```python
from build123d import *

# Parameters (mm, degrees)
SKETCH1_W                       = 180
SKETCH1_H                       = 60
BOSS_EXTRUDE1_DEPTH             = 15
CUT_EXTRUDE1_DEPTH              = 97.046863561
TAP_DRILL_FOR_M6X1_0_TAP1_D     = 5
TAP_DRILL_FOR_M6X1_0_TAP1_DEPTH = 9
TAP_DRILL_FOR_M6X1_0_TAP1_TIP   = 1.502151548
FILLET1_R                       = 25
TAP_DRILL_FOR_M6X1_0_TAP2_D     = 5
TAP_DRILL_FOR_M6X1_0_TAP2_DEPTH = 9
TAP_DRILL_FOR_M6X1_0_TAP2_TIP   = 1.502151548


with BuildPart() as part:
    # Sketch1 → Boss-Extrude1 (new body)
    with BuildSketch(Plane(origin=(0, 0, 0), x_dir=(1, 0, 0), z_dir=(0, 1, 0))):
        Rectangle(SKETCH1_W, SKETCH1_H)
    extrude(amount=BOSS_EXTRUDE1_DEPTH)

    # Sketch2 → Cut-Extrude1 (cut, through all)
    with BuildSketch(Plane(origin=(0, 15, 0), x_dir=(1, 0, 0), z_dir=(0, 1, 0))):
        with BuildLine():
            Line((-60, 17.5), (-23.75, 17.5))
            ThreePointArc((-23.75, 17.5), (-6.25, 0), (-23.75, -17.5))
            Line((-23.75, -17.5), (-60, -17.5))
            ThreePointArc((-60, -17.5), (-77.5, 0), (-60, 17.5))
        make_face()
        with BuildLine():
            Line((23.75, 17.5), (60, 17.5))
            ThreePointArc((60, 17.5), (77.5, 0), (60, -17.5))
            Line((60, -17.5), (23.75, -17.5))
            ThreePointArc((23.75, -17.5), (6.25, 0), (23.75, 17.5))
        make_face()
    extrude(amount=-CUT_EXTRUDE1_DEPTH, mode=Mode.SUBTRACT)

    # Tap Drill for M6x1.0 Tap1
    with Locations(Plane.XY.offset(30)):
        with Locations((60, 7.5), (-20, 7.5), (20, 7.5), (-60, 7.5)):
            Hole(TAP_DRILL_FOR_M6X1_0_TAP1_D / 2, depth=TAP_DRILL_FOR_M6X1_0_TAP1_DEPTH)
            with Locations((0, 0, -(TAP_DRILL_FOR_M6X1_0_TAP1_DEPTH + TAP_DRILL_FOR_M6X1_0_TAP1_TIP / 2))):  # 118° drill point
                Cone(0, TAP_DRILL_FOR_M6X1_0_TAP1_D / 2, TAP_DRILL_FOR_M6X1_0_TAP1_TIP, mode=Mode.SUBTRACT)

    # Fillet1
    fillet1_edges = [part.edges().sort_by_distance(p)[0] for p in [
        (-90, 7.5, -30),
        (90, 7.5, -30),
    ]]
    fillet(fillet1_edges, radius=FILLET1_R)

    # Tap Drill for M6x1.0 Tap2
    with Locations(Plane(origin=(0, 0, -30), x_dir=(-1, 0, 0), z_dir=(0, 0, -1))):
        with Locations((-45, 7.5), (-15, 7.5), (15, 7.5), (45, 7.5)):
            Hole(TAP_DRILL_FOR_M6X1_0_TAP2_D / 2, depth=TAP_DRILL_FOR_M6X1_0_TAP2_DEPTH)
            with Locations((0, 0, -(TAP_DRILL_FOR_M6X1_0_TAP2_DEPTH + TAP_DRILL_FOR_M6X1_0_TAP2_TIP / 2))):  # 118° drill point
                Cone(0, TAP_DRILL_FOR_M6X1_0_TAP2_D / 2, TAP_DRILL_FOR_M6X1_0_TAP2_TIP, mode=Mode.SUBTRACT)


solid = part.part
```
Read the model definition and answer for the solid it produces. Units are mm, in the model's axes. A direction names the side the tool comes from. Round coordinates to 2 decimals unless told otherwise and drop trailing zeros. Write each loop counter-clockwise with the first axis right and the second up, starting at its lowest first coordinate (ties: lowest second). Pieces come first, ordered by that corner, then holes. Notation, with made-up numbers: (33, 67) - (91, 67) arc R17 cw to (91, 84) - close; hole circle Ø6 at (-12.5, -38). An arc over 180 degrees is marked (long way). One line per item, written item: value.
Q1. For a pull along Y with two mould halves and no side action, classify faces 1 (the flat face through (-1, 15, 0)), 2 (the cylindrical face through (57.69, 6.54, 25.44)), 3 (the flat face through (-1, 7, -30)) as pulls with the +Y half, pulls with the -Y half, needs draft (parallel to the pull), parting line crosses it, or undercut.
The answers:
face 1: pulls with the +Y half
face 2: undercut
face 3: needs draft
Q2. Straight lines are drawn through the part: line 1 (X direction, y = 6, z = -1); line 2 (Z direction, x = -42.5, y = 1.75); line 3 (Y direction, x = -15, z = -23.75). For each, find the intervals that lie inside material, in ascending order. Write a range as from..to.
The answers:
line 1: x = -90..-77.47, -6.28..6.28, 77.47..90
line 2: z = -30..-17.5, 17.5..30
line 3: y = 0..5, 10..15
Q3. Find section C-C (x = -69). Determine the outline of the cut face in (y, z), and give its area (3 significant figures).
The answers:
outline: (0, -29.68) - (15, -29.68) - (15, -15.01) - (0, -15.01) - close; (0, 15.01) - (15, 15.01) - (15, 30) - (0, 30) - close
area: 445 mm2
Q4. Which of the six approach directions +Z, -Z, +X, -X, +Y, -Y give full straight-line access (tool end or side, diameter ignored) to faces 4 (the flat face through (-42, 8, 17.5)), 5 (the cylindrical face through (-18, 6, 25)), 6 (the cylindrical face through (-82.871, 7.605, -22.482)), 7 (the cylindrical face through (13, 6, -25))?
The answers:
face 4: +Y, -Y
face 5: +Z
face 6: -Z, -X, +Y, -Y
face 7: -Z
Q5. Find section B-B (z = 0). Determine the outline of the cut face in (x, y).
The answers:
outline: (-90, 0) - (-77.5, 0) - (-77.5, 15) - (-90, 15) - close; (-6.25, 0) - (6.25, 0) - (6.25, 15) - (-6.25, 15) - close; (77.5, 0) - (90, 0) - (90, 15) - (77.5, 15) - close
Q6. Each of these flat-tipped pins is pushed along its axis until it touches: P1, Ø2, axis at y = 13, z = -12.5, coming from the -X side; P2, Ø1.5, axis at y = 11, z = -7, coming from the +X side; P3, Ø3, axis at x = 45, y = 7.5, coming from the -Z side. Where does it stop, or does it pass through?
The answers:
P1: stops at x = -89.14
P2: stops at x = 89.97
P3: stops at z = -20.4
Q7. Find section A-A (x = 51.5). Determine the outline of the cut face in (y, z).
The answers:
outline: (0, -30) - (15, -30) - (15, -17.5) - (0, -17.5) - close; (0, 17.5) - (15, 17.5) - (15, 30) - (0, 30) - close
